```python
from build123d import *

# Parameters (mm, degrees)
RAO_OUTLET_RADIUS_R     = 2.742884532
F_1_4_CLEARANCE_HOLE1_D = 6.7564
SKETCH5_OUTSIDE_W       = 174.362
SKETCH5_OUTSIDE_H       = 174.362
SKETCH5_OUTSIDE_R       = 45.72
CUT_EXTRUDE1_DEPTH      = 5.08
FILLET1_R               = 3.175
RAO_INLET_RADIUS_R      = 10.770489


with BuildPart() as part:
    # Sketch1 → Nozzle (revolve)
    with BuildSketch(Plane.XY):
        Polygon((15.288121734, 7.180326), (21.511121734, 7.180326), (38.957805968, 11.855150951), (38.957805968, 27.500000118), (5.08, 27.500000118), (5.08, 66.870000118), (0, 66.870000118), (0, 25.4), align=None)
    revolve(axis=Axis((0, 0, 0), (1, 0, 0)))

    # Rao outlet radius
    rao_outlet_radius_edges = [part.edges().sort_by_distance(p)[0] for p in [
        (21.511121734, -7.180326, 0),
    ]]
    fillet(rao_outlet_radius_edges, radius=RAO_OUTLET_RADIUS_R)

    # 1/4 Clearance Hole1 (through all)
    with Locations(Plane.ZY):
        with Locations((37.465, 0), (26.491755557, -26.491755557), (0, -37.465), (-26.491755557, -26.491755557), (-37.465, 0), (-26.491755557, 26.491755557), (0, 37.465), (26.491755557, 26.491755557), (0, 0)):
            Hole(F_1_4_CLEARANCE_HOLE1_D / 2)

    # Sketch5 outside → Cut-Extrude1 (cut)
    with BuildSketch(Plane(origin=(0, 0, 0), x_dir=(0, 0, -1), z_dir=(1, 0, 0))):
        Rectangle(SKETCH5_OUTSIDE_W, SKETCH5_OUTSIDE_H)
        Circle(SKETCH5_OUTSIDE_R, mode=Mode.SUBTRACT)
    extrude(amount=CUT_EXTRUDE1_DEPTH, mode=Mode.SUBTRACT)

    # Fillet1
    fillet1_edges = [part.edges().sort_by_distance(p)[0] for p in [
        (5.08, -27.500000118, 0),
    ]]
    fillet(fillet1_edges, radius=FILLET1_R)

    # Rao Inlet radius
    rao_inlet_radius_edges = [part.edges().sort_by_distance(p)[0] for p in [
        (15.288121734, -7.180326, 0),
    ]]
    fillet(rao_inlet_radius_edges, radius=RAO_INLET_RADIUS_R)


solid = part.part
```
For this review, take the finished solid that the model builds, in its own axes (mm). A direction names the side the tool comes from. Coordinates: 2 decimals unless noted, no trailing zeros. Write each loop counter-clockwise with the first axis right and the second up, starting at its lowest first coordinate (ties: lowest second). Pieces come first, ordered by that corner, then holes. Notation, with made-up numbers: (20.5, 52) - (71.5, 52) arc R28 cw to (71.5, 76) - close; hole circle Ø7 at (71.25, 5). An arc over 180 degrees is marked (long way). Answer in a Markdown table with one row per item. Add a question column.
Q1. We need section B-B, the plane z = 0. Count the separate pieces of the cut face and the enclosed holes in it, and give its area (3 significant figures).
Q2. We need section D-D, the plane x = 34. State the section outline as (y, z) points, and give its area (3 significant figures).
Q3. For probe 1 along Z at (x, y) = (20.75, 0); probe 2 along Y at (x, z) = (30, -1); probe 3 along Y at (x, z) = (12, 1), list the stretches that pass through material, from the lowest coordinate up.
Q4. Draft analysis for pull direction Y (two halves, no side actions). For faces 3 (the cylindrical face through (2.58, -29.79, 27.22)), 4 (the flat face through (5.08, 1, 31)), 5 (the cylindrical face through (2.5, 13.73, -43.61)), state which applies: +Y half, -Y half, draft (parallel to the pull), parting line (faces both ways), or undercut.
Q5. For P1, Ø1, axis at y = -27.5, z = 34, coming from the +X side; P2, Ø2, axis at y = 9.5, z = -8, coming from the -X side; P3, Ø3, axis at x = 30.5, y = -7.5, coming from the +Z side, all flat-tipped, find the tip position at first contact; note any pin that passes through.
Q6. We need section A-A, the plane z = -38.5. State the section outline as (x, y) points, and give its area (3 significant figures).
Q7. Tool access review of faces 1 (the cylindrical face through (2.58, 0.15, -34.09)), 2 (the cylindrical face through (23.391, -5.961, -26.846)): name each direction out of +Z, -Z, +X, -X, +Y, -Y from which nothing blocks a thin tool from reaching the whole face with its end or side.
Answer list:
| question | item | result |
|---|---|---|
| 1 | separate pieces | 4 |
| 1 | enclosed holes | 0 |
| 1 | area | 1,340 mm2 |
| 2 | outline | circle Ø55 at (0, 0); hole circle Ø21.05 at (0, 0) |
| 2 | area | 2,030 mm2 |
| 3 | probe 1 | z = -27.5 to -7.18, 7.18 to 27.5 |
| 3 | probe 2 | y = -27.48 to -9.4, 9.4 to 27.48 |
| 3 | probe 3 | y = -27.48 to -11.05, 11.05 to 27.48 |
| 4 | face 3 | undercut |
| 4 | face 4 | draft |
| 4 | face 5 | parting line |
| 5 | P1 | stops at x = 5.08 |
| 5 | P2 | stops at x = 10.05 |
| 5 | P3 | stops at z = 26.84 |
| 6 | outline | (0, -24.66) - (5.08, -24.66) - (5.08, -3.22) - (0, -3.22) - close; (0, 3.22) - (5.08, 3.22) - (5.08, 24.66) - (0, 24.66) - close |
| 6 | area | 218 mm2 |
| 7 | face 1 | +X, -X |
| 7 | face 2 | +X |
